```python
from build123d import *

# Parameters (mm, degrees)
F0_R     = 11.08075
F1_DEPTH = 6.35


with BuildPart() as f1:
    # F0 (on Front) → F1 (new body)
    with BuildSketch(Plane.XZ):
        with BuildLine():
            ThreePointArc((0, -11.08075), (-11.08075, 0), (0, 11.08075))
            Line((0, 11.08075), (0, 11.43))
            ThreePointArc((0, 11.43), (-2.9784140075, 11.7511923598), (-5.8198711326, 12.7))
            ThreePointArc((-5.8198711326, 12.7), (-9.4037860849, 10.3310070791), (-12.0983749873, 6.9849998329))
            ThreePointArc((-12.0983749873, 6.9849998329), (-13.6488076608, 2.9784139133), (-13.9084581944, -1.3098437524))
            ThreePointArc((-13.9084581944, -1.3098437524), (-9.8986703653, -5.715), (-8.0885870618, -11.3901562476))
            ThreePointArc((-8.0885870618, -11.3901562476), (-4.2450216288, -13.3094211509), (-4.4e-09, -13.97))
            Line((0, -13.97), (0, -11.08075))
        make_face()
        with BuildLine():
            ThreePointArc((-13.9084581944, -1.3098437524), (-12.0983748909, -6.985), (-8.0885870618, -11.3901562476))
            ThreePointArc((-8.0885870618, -11.3901562476), (-9.8986703653, -5.715), (-13.9084581944, -1.3098437524))
        make_face()
        with BuildLine():
            ThreePointArc((-8.0270452561, -12.7), (-8.042439189, -12.044355651), (-8.0885870618, -11.3901562476))
            ThreePointArc((-8.0885870618, -11.3901562476), (-12.0983748909, -6.985), (-13.9084581944, -1.3098437524))
            ThreePointArc((-13.9084581944, -1.3098437524), (-17.7520236295, 0.6094211516), (-21.9970452561, 1.27))
            ThreePointArc((-21.9970452561, 1.27), (-34.095420147, -19.685), (-9.8986703653, -19.685))
            ThreePointArc((-9.8986703653, -19.685), (-8.5030614629, -16.3157020601), (-8.0270452561, -12.7))
        make_face()
        with Locations((-21.9970452561, -12.7)):
            Circle(F0_R, mode=Mode.SUBTRACT)
        with BuildLine():
            ThreePointArc((-13.9084581944, -1.3098437524), (-13.6488076608, 2.9784139133), (-12.0983749873, 6.9849998329))
            ThreePointArc((-12.0983749873, 6.9849998329), (-16.2820453397, 2.8013295865), (-21.9970452561, 1.27))
            ThreePointArc((-21.9970452561, 1.27), (-17.7520236295, 0.6094211516), (-13.9084581944, -1.3098437524))
        make_face()
        with BuildLine():
            ThreePointArc((-12.0983749873, 6.9849998329), (-9.4037860849, 10.3310070791), (-5.8198711326, 12.7))
            ThreePointArc((-5.8198711326, 12.7), (-9.4037860136, 15.0689928559), (-12.0983748909, 18.415))
            ThreePointArc((-12.0983748909, 18.415), (-10.5670452561, 12.6999999036), (-12.0983749873, 6.9849998329))
        make_face()
        with BuildLine():
            ThreePointArc((-5.8198711326, 12.7), (-2.9784140075, 13.6488076402), (0, 13.97))
            ThreePointArc((0, 13.97), (2.9784140075, 13.6488076402), (5.8198711326, 12.7))
            ThreePointArc((5.8198711326, 12.7), (9.4037860136, 15.0689928559), (12.0983748909, 18.415))
            ThreePointArc((12.0983748909, 18.415), (13.4939837933, 21.7842979399), (13.97, 25.4))
            ThreePointArc((13.97, 25.4), (-3.6157020601, 38.8939837933), (-12.0983748909, 18.415))
            ThreePointArc((-12.0983748909, 18.415), (-9.4037860136, 15.0689928559), (-5.8198711326, 12.7))
        make_face()
        with BuildLine():
            ThreePointArc((11.08075, 25.4), (7.8352734656, 17.5647265344), (0, 14.31925))
            ThreePointArc((0, 14.31925), (-7.8352734656, 33.2352734656), (11.08075, 25.4))
        make_face(mode=Mode.SUBTRACT)
        with BuildLine():
            ThreePointArc((-5.8198711326, 12.7), (-2.9784140075, 11.7511923598), (0, 11.43))
            Line((0, 11.43), (0, 13.97))
            ThreePointArc((0, 13.97), (-2.9784140075, 13.6488076402), (-5.8198711326, 12.7))
        make_face()
        with BuildLine():
            Line((0, 13.97), (0, 11.43))
            ThreePointArc((0, 11.43), (2.9784140075, 11.7511923598), (5.8198711326, 12.7))
            ThreePointArc((5.8198711326, 12.7), (2.9784140075, 13.6488076402), (0, 13.97))
        make_face()
        with BuildLine():
            ThreePointArc((0, 11.08075), (7.8352734656, 7.8352734656), (11.08075, 0))
            ThreePointArc((11.08075, 0), (7.8352734656, -7.8352734656), (0, -11.08075))
            Line((0, -11.08075), (0, -13.97))
            ThreePointArc((-4.4e-09, -13.97), (4.2450216245, -13.3094211522), (8.0885870618, -11.3901562476))
            ThreePointArc((8.0885870618, -11.3901562476), (9.8986703653, -5.715), (13.9084581944, -1.3098437524))
            ThreePointArc((13.9084581944, -1.3098437524), (13.9546060671, -0.655644349), (13.97, 0))
            ThreePointArc((13.97, 0), (13.4939837983, 3.6157020414), (12.0983749102, 6.9849999665))
            ThreePointArc((12.0983749102, 6.9849999665), (9.4037860279, 10.331007131), (5.8198711326, 12.7))
            ThreePointArc((5.8198711326, 12.7), (2.9784140075, 11.7511923598), (0, 11.43))
            Line((0, 11.43), (0, 11.08075))
        make_face()
        with BuildLine():
            ThreePointArc((12.0983748909, 18.415), (9.4037860136, 15.0689928559), (5.8198711326, 12.7))
            ThreePointArc((5.8198711326, 12.7), (9.4037860279, 10.331007131), (12.0983749102, 6.9849999665))
            ThreePointArc((12.0983749102, 6.9849999665), (10.5670452561, 12.6999999806), (12.0983748909, 18.415))
        make_face()
        with BuildLine():
            ThreePointArc((21.9970452561, 1.27), (16.2820452729, 2.8013296251), (12.0983749102, 6.9849999665))
            ThreePointArc((12.0983749102, 6.9849999665), (13.4939837983, 3.6157020414), (13.97, 0))
            ThreePointArc((13.97, 0), (13.9546060671, -0.655644349), (13.9084581944, -1.3098437524))
            ThreePointArc((13.9084581944, -1.3098437524), (17.7520236295, 0.6094211516), (21.9970452561, 1.27))
        make_face()
        with BuildLine():
            ThreePointArc((13.9084581944, -1.3098437524), (12.0983748909, -6.985), (8.0885870618, -11.3901562476))
            ThreePointArc((8.0885870618, -11.3901562476), (8.3482376159, -15.6784140075), (9.8986703653, -19.685))
            ThreePointArc((9.8986703653, -19.685), (25.6127473162, -26.1939837933), (35.9670452561, -12.7))
            ThreePointArc((35.9670452561, -12.7), (31.8753269893, -2.8217182668), (21.9970452561, 1.27))
            ThreePointArc((21.9970452561, 1.27), (17.7520236295, 0.6094211516), (13.9084581944, -1.3098437524))
        make_face()
        with Locations((21.9970452561, -12.7)):
            Circle(F0_R, mode=Mode.SUBTRACT)
        with BuildLine():
            ThreePointArc((13.9084581944, -1.3098437524), (9.8986703653, -5.715), (8.0885870618, -11.3901562476))
            ThreePointArc((8.0885870618, -11.3901562476), (12.0983748909, -6.985), (13.9084581944, -1.3098437524))
        make_face()
        with BuildLine():
            ThreePointArc((-9.8986703653, -19.685), (-5.7150000019, -15.5013296359), (-4.4e-09, -13.97))
            ThreePointArc((-4.4e-09, -13.97), (-4.2450216288, -13.3094211509), (-8.0885870618, -11.3901562476))
            ThreePointArc((-8.0885870618, -11.3901562476), (-8.042439189, -12.044355651), (-8.0270452561, -12.7))
            ThreePointArc((-8.0270452561, -12.7), (-8.5030614629, -16.3157020601), (-9.8986703653, -19.685))
        make_face()
        with BuildLine():
            ThreePointArc((8.0885870618, -11.3901562476), (4.2450216245, -13.3094211522), (-4.4e-09, -13.97))
            ThreePointArc((-4.4e-09, -13.97), (5.7149999981, -15.5013296336), (9.8986703653, -19.685))
            ThreePointArc((9.8986703653, -19.685), (8.3482376159, -15.6784140075), (8.0885870618, -11.3901562476))
        make_face()
    extrude(amount=F1_DEPTH)


solid = f1.part
```
Build history of the part. All positions in model axes, mm. Coordinates: 2 decimals unless noted, no trailing zeros. Order: outer loops, then holes, each group sorted by start corner. A loop starts at its lowest first (then second) coordinate and runs counter-clockwise, first axis right, second up.
Item 1: Saw through at B-B on x = -30. List the corners of the cut face in (y, z).
Filled in:
outline: (-6.35, -24.15) - (0, -24.15) - (0, -20.36) - (-6.35, -20.36) - close; (-6.35, -5.04) - (0, -5.04) - (0, -1.25) - (-6.35, -1.25) - close
Item 2: Saw through at C-C on x = 6. List the corners of the cut face in (y, z).
Filled in:
outline: (-6.35, -15.67) - (0, -15.67) - (0, -9.32) - (-6.35, -9.32) - close; (-6.35, 9.32) - (0, 9.32) - (0, 16.08) - (-6.35, 16.08) - close; (-6.35, 34.72) - (0, 34.72) - (0, 38.02) - (-6.35, 38.02) - close
Item 3: Drop flat-ended pins along their axis: pin 1 Ø3 at (y, z) = (-0.5, 29) entering from -X; pin 2 Ø13.5 at (x, z) = (-22, -12.7) entering from +Y; pin 3 Ø1.5 at (y, z) = (-4, 15) entering from -X; pin 4 Ø1.5 at (x, y) = (-7.5, -3) entering from +Z. Give the stop position or say it passes through.
Filled in:
pin 1: stops at x = -13.81
pin 2: passes through
pin 3: stops at x = -10.98
pin 4: stops at z = 37.63
Item 4: Saw through at D-D on x = -18.5. List the corners of the cut face in (y, z), then the cut area to 3 significant figures.
Filled in:
outline: (-6.35, -26.23) - (0, -26.23) - (0, -23.21) - (-6.35, -23.21) - close; (-6.35, -2.19) - (0, -2.19) - (0, 1.82) - (-6.35, 1.82) - close
area: 44.5 mm2
Item 5: Mould opens along X. For faces 1 (the flat face through (-0.2, 0, 11.4)), 2 (the cylindrical face through (-11.43, -3.13, -9.37)) say: released by +X, released by -X, zero draft, split by the parting line, or undercut.
Filled in:
face 1: zero draft
face 2: undercut
Item 6: Saw through at A-A on y = -5. List the corners of the cut face in (x, z) (1 decimal), then the cut area to 3 significant figures.
Filled in:
outline: (-22, 1.3) arc R14 ccw (long way) to (-9.9, -19.7) arc R11.4 cw to (9.9, -19.7) arc R14 ccw (long way) to (22, 1.3) arc R11.4 cw to (12.1, 18.4) arc R14 ccw (long way) to (-12.1, 18.4) arc R11.4 cw to start; hole circle Ø22.2 at (-22, -12.7); hole circle Ø22.2 at (0, 0); hole circle Ø22.2 at (0, 25.4); hole circle Ø22.2 at (22, -12.7)
area: 949 mm2
Item 7: Drill centre lines: L1, parallel to X at y = -6, z = -4; L2, parallel to Z at x = -4, y = -2.5; L3, parallel to Z at x = -12, y = -0.75. Where is each one in solid material? Low to high.
Filled in:
L1: x = -32.93 to -28.86, -15.13 to -10.33, 10.33 to 15.13, 28.86 to 32.93
L2: z = -14.69 to -10.33, 10.33 to 15.07, 35.73 to 38.79
L3: z = -22.46 to -17.48, -7.92 to 7.16, 18.24 to 32.55
